Could you check a few things on this drawing? It's one solid part, dimensions in mm from its lowest x, y, z. Round coordinates to 2 decimals unless told otherwise and drop trailing zeros. Loops run counter-clockwise (first coordinate to the right, second up) from the corner with the lowest first, then second, coordinate; pieces in that order, holes last. Notation, with made-up numbers: M -38,-14 L -17,-14 A25 ccw -17,20 Z; hole C 13,85.5 d4. An arc over 180 degrees is marked long. Return JSON: item names as keys, results as strings.
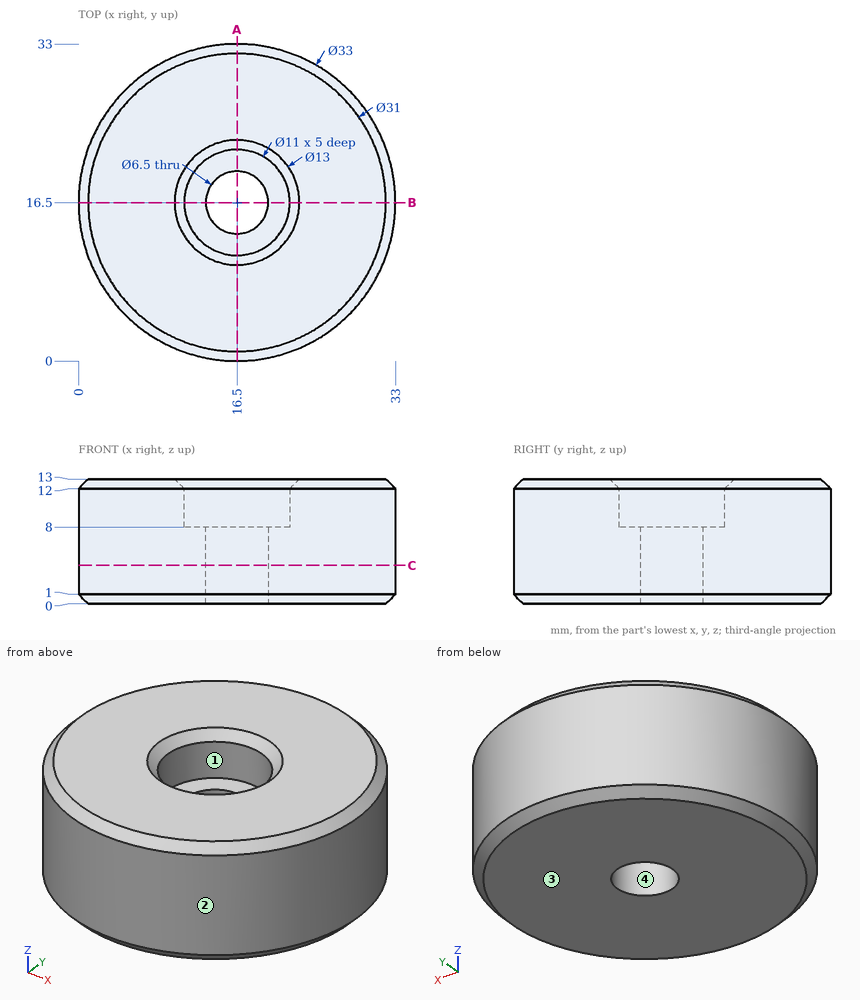
Q1. If I drill on line 1 along Y through (x, z) = (16.5, 5); line 2 along Y through (x, z) = (16.5, 9.5); line 3 along Z through (x, y) = (20, 12.5), over which ranges is the centre line in solid material (lowest first)?
Results:
{"line 1": "y = 0 to 13.25, 19.75 to 33", "line 2": "y = 0 to 11, 22 to 33", "line 3": "z = 0 to 8"}
Q2. Suppose I cut it at A-A, the plane x = 16.5. Please give me the cut outline in (y, z).
Results:
{"outline": "M 0,1 L 1,0 L 13.25,0 L 13.25,8 L 11,8 L 11,12 L 10,13 L 1,13 L 0,12 Z; M 19.75,0 L 32,0 L 33,1 L 33,12 L 32,13 L 23,13 L 22,12 L 22,8 L 19.75,8 Z"}
Q3. Suppose I cut it at C-C, the plane z = 4. Please give me the cut outline in (x, y), plus the area to 3 significant figures.
Results:
{"outline": "C 16.5,16.5 d33; hole C 16.5,16.5 d6.5", "area": "822 mm2"}
Q4. Thinking about a two-plate mould opening in X: for the marked faces 1, 2, 3 and 4, which applies, pulls with the +X half, pulls with the -X half, needs draft (parallel to the pull), parting line crosses it, or undercut?
Results:
{"face 1": "undercut", "face 2": "parting line crosses it", "face 3": "needs draft", "face 4": "undercut"}
Q5. I'm going to push flat-ended pins straight in: pin 1 Ø4 at (x, y) = (16.5, 16.5) entering from +Z; pin 2 Ø2 at (y, z) = (14, 6) entering from -X; pin 3 Ø1.5 at (x, z) = (4.5, 3) entering from -Y; pin 4 Ø1.5 at (x, z) = (12, 3.5) entering from -Y. Where does each tip first touch, or does it pass through?
Results:
{"pin 1": "passes through", "pin 2": "stops at x = 0.07", "pin 3": "stops at y = 4.43", "pin 4": "stops at y = 0.43"}
